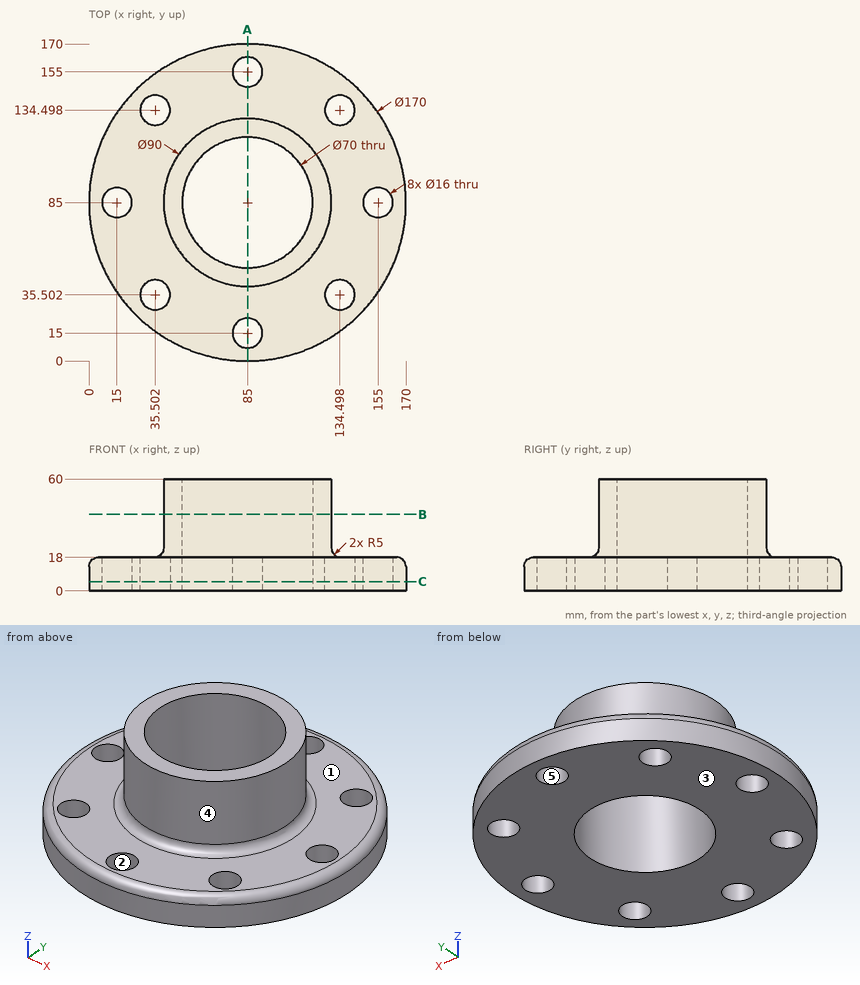
Can you work these out from the drawing? Everything is in mm from the part's minimum corner. A direction names the side the tool comes from. Round coordinates to 2 decimals unless told otherwise and drop trailing zeros. Loops run counter-clockwise (first coordinate to the right, second up) from the corner with the lowest first, then second, coordinate; pieces in that order, holes last. Notation, with made-up numbers: M 4,19.5 L 63,19.5 A17 ccw 63,42.5 Z; hole C 64.5,76 d7. An arc over 180 degrees is marked long. Write item = value, one per line.
1. Which directions (+Z, -Z, +X, -X, +Y, -Y) give clear straight access to the entire face, cutting with the end or side of a thin tool? Please do the marked faces 1 and 2.
Results below:
face_1 = +Z
face_2 = +Z, -Z
2. I want a section at B-B, the plane z = 41. Write out the boundary of the cut face in (x, y), and give its area (3 significant figures).
Results below:
outline = C 85,85 d90; hole C 85,85 d70
area = 2,510 mm²
3. Will these pins go through, and if not, where does the flat tip stop? P1, Ø5, axis at x = 113, y = 137, coming from the -Z side; P2, Ø12, axis at x = 151.5, y = 61.5, coming from the +Z side; P3, Ø12, axis at y = 83, z = 19.5, coming from the -X side; P4, Ø12, axis at x = 128.5, z = 48, coming from the +Y side (1 decimal).
Results below:
P1 = 0
P2 = 18
P3 = 0.04
P4 = 109.9
4. I want a section at A-A, the plane x = 85. Write out the boundary of the cut face in (y, z), and give its area (3 significant figures).
Results below:
outline = M 0,0 L 7,0 L 7,18 L 5,18 A5 ccw 0,13 Z; M 23,0 L 50,0 L 50,60 L 40,60 L 40,23 A5 cw 35,18 L 23,18 Z; M 120,0 L 147,0 L 147,18 L 135,18 A5 cw 130,23 L 130,60 L 120,60 Z; M 163,0 L 170,0 L 170,13 A5 ccw 165,18 L 163,18 Z
area = 2,060 mm²
5. Thinking about a two-plate mould opening in X: for the marked faces 3, 4 and 5, which applies, +X half, -X half, draft (parallel to the pull), parting line (faces both ways), or undercut?
Results below:
face_3 = draft
face_4 = parting line
face_5 = undercut
6. I need wall thicknesses on probe 1 along X at (y, z) = (42.5, 3) (1 decimal); probe 2 along Z at (x, y) = (160, 99); probe 3 along X at (y, z) = (30, 16) (1 decimal). Which ranges of each line are inside material? Lowest first, please.
Results below:
probe_1 = 11.4 to 31.6, 39.4 to 130.6, 138.4 to 158.6
probe_2 = 0 to 18
probe_3 = 21.5 to 29.7, 41.3 to 128.7, 140.3 to 148.5
7. I want a section at C-C, the plane z = 5. Count the separate pieces of the cut face and the enclosed holes in it, and give its area (3 significant figures).
Results below:
separate_pieces = 1
enclosed_holes = 9
area = 17,200 mm²
